```python
from build123d import *

# Parameters (mm, degrees)
SKETCH1_R           = 7.5
BOSS_EXTRUDE1_DEPTH = 24
SKETCH2_R           = 1.75
CUT_EXTRUDE1_DEPTH  = 24
CUT_EXTRUDE2_START  = -10
CUT_EXTRUDE2_DEPTH  = 7


with BuildPart() as part:
    # Sketch1 → Boss-Extrude1 (new body)
    with BuildSketch(Plane.XY):
        Polygon((0, 10), (0, 0), (-10, -10), (-20, -10), (-30, 0), (-30, 10), align=None)
        with Locations((-15, 0)):
            Circle(SKETCH1_R, mode=Mode.SUBTRACT)
    extrude(amount=BOSS_EXTRUDE1_DEPTH)

    # Sketch2 → Cut-Extrude1 (cut)
    with BuildSketch(Plane(origin=(0, 10, 0), x_dir=(1, 0, 0), z_dir=(0, 1, 0))):
        with Locations((-26.5, -12)):
            Circle(SKETCH2_R)
        with Locations((-3.5, -12)):
            Circle(SKETCH2_R)
    extrude(amount=-CUT_EXTRUDE1_DEPTH, mode=Mode.SUBTRACT)

    # Sketch4 → Cut-Extrude2 (cut)
    with BuildSketch(Plane(origin=(0, 10, 0), x_dir=(1, 0, 0), z_dir=(0, 1, 0)).offset(CUT_EXTRUDE2_START)):
        Polygon((-3.5, -15.175426481), (-0.75, -13.58771324), (-0.75, -10.41228676), (-3.5, -8.824573519), (-6.25, -10.41228676), (-6.25, -13.58771324), align=None)
        Polygon((-26.5, -15.175426481), (-23.75, -13.58771324), (-23.75, -10.41228676), (-26.5, -8.824573519), (-29.25, -10.41228676), (-29.25, -13.58771324), align=None)
    extrude(amount=-CUT_EXTRUDE2_DEPTH, mode=Mode.SUBTRACT)


solid = part.part
```
Work out the finished part from the listing and answer in its coordinate system (mm). A direction names the side the tool comes from. Give positions to 0.01 mm unless a question says otherwise; leave off trailing zeros. Loops run counter-clockwise (first coordinate to the right, second up) from the corner with the lowest first, then second, coordinate; pieces in that order, holes last. Notation, with made-up numbers: M 38.25,65.25 L 84.25,65.25 A14 cw 84.25,84.25 Z; hole C -30.5,-21 d3. An arc over 180 degrees is marked long. One line per item, written item: value. Start each with the question number.
1. Which of the six approach directions +Z, -Z, +X, -X, +Y, -Y give full straight-line access (tool end or side, diameter ignored) to faces 1 (the face through (-4.86, -2.39, 9.61)), 2 (the face through (-11, 7, 0))?
2. Find section B-B (y = 6.5). Give the vertices of the cut face in (x, z), and give its area (3 significant figures).
3. Find the intervals of material crossed by probe 1 along Z at (x, y) = (-3.5, 7); probe 2 along X at (y, z) = (2.5, 12); probe 3 along Y at (x, z) = (-8.5, 6.75), in increasing order.
4. Find section D-D (z = 7.25). Give the vertices of the cut face in (x, y).
5. Each of these flat-tipped pins is pushed along its axis until it touches: P1, Ø4, axis at y = 6.5, z = 15, coming from the +X side; P2, Ø4, axis at y = -2.5, z = 8, coming from the +X side; P3, Ø3, axis at x = -6, z = 14.5, coming from the -Y side; P4, Ø3, axis at y = -4.5, z = 17, coming from the +X side. Where does it stop, or does it pass through?
6. Find section A-A (z = 12). Give the vertices of the cut face in (x, y), and give its area (3 significant figures).
7. Find section C-C (x = -15). Give the vertices of the cut face in (y, z).
8. Determine the mould class of faces 3 (the face through (-3.728, 5.07, 10.265)), 4 (the face through (-4.8, 0, 13.4)), 5 (the face through (-11, 7, 24)), 6 (the face through (-25, -5, 9)) for opening direction Z: released by +Z, released by -Z, zero draft, split by the parting line, or undercut.
Reported:
1. face 1: -Y
1. face 2: -Z, +X, -X, +Y, -Y
2. outline: M -30,0 L -18.74,0 L -18.74,24 L -30,24 Z; M -11.26,0 L 0,0 L 0,24 L -11.26,24 Z; hole C -26.5,12 d3.5; hole C -3.5,12 d3.5
2. area: 521 mm²
3. probe 1: z = 0 to 10.25, 13.75 to 24
3. probe 2: x = -30 to -28.25, -24.75 to -22.07, -7.93 to -5.25, -1.75 to 0
3. probe 3: y = -8.5 to -3.74, 3.74 to 10
4. outline: M -30,0 L -20,-10 L -10,-10 L 0,0 L 0,10 L -30,10 Z; hole C -15,0 d15
5. P1: stops at x = 0
5. P2: stops at x = -0.5
5. P3: stops at y = -7.5
5. P4: stops at x = -3
6. outline: M -30,0 L -29.25,-0.75 L -29.25,0 L -28.25,0 L -28.25,10 L -30,10 Z; M -24.75,0 L -23.75,0 L -23.75,-6.25 L -20,-10 L -10,-10 L -6.25,-6.25 L -6.25,0 L -5.25,0 L -5.25,10 L -24.75,10 Z; M -1.75,0 L -0.75,0 L -0.75,-0.75 L 0,0 L 0,10 L -1.75,10 Z; hole C -15,0 d15
6. area: 215 mm²
7. outline: M -10,0 L -7.5,0 L -7.5,24 L -10,24 Z; M 7.5,0 L 10,0 L 10,24 L 7.5,24 Z
8. face 3: undercut
8. face 4: undercut
8. face 5: released by +Z
8. face 6: zero draft
